from build123d import *

# Parameters (mm, degrees)
SKETCH1_W           = 7
SKETCH1_H           = 7
BOSS_EXTRUDE1_DEPTH = 3
FILLET1_R           = 1
BOSS_EXTRUDE2_DEPTH = 0.2
FILLET2_R           = 0.2


with BuildPart() as part:
    # Sketch1 → Boss-Extrude1 (new body)
    with BuildSketch(Plane(origin=(0, 0, 0), x_dir=(1, 0, 0), z_dir=(0, 1, 0))):
        Rectangle(SKETCH1_W, SKETCH1_H)
    extrude(amount=BOSS_EXTRUDE1_DEPTH)

    # Fillet1
    fillet1_edges = [part.edges().sort_by_distance(p)[0] for p in [
        (-3.5, 3, 0),
        (0, 3, 3.5),
        (3.5, 3, 0),
        (0, 3, -3.5),
        (3.5, 1.5, 3.5),
        (-3.5, 1.5, 3.5),
        (-3.5, 1.5, -3.5),
        (3.5, 1.5, -3.5),
    ]]
    fillet(fillet1_edges, radius=FILLET1_R)

    # Sketch2 → Boss-Extrude2 (add)
    with BuildSketch(Plane(origin=(0, 3, 0), x_dir=(1, 0, 0), z_dir=(0, 1, 0))):
        Polygon((0, 2), (-1.732050808, -1), (1.732050808, -1), align=None)
    extrude(amount=BOSS_EXTRUDE2_DEPTH)

    # Fillet2
    fillet2_edges = [part.edges().sort_by_distance(p)[0] for p in [
        (-0.866025404, 3.2, -0.5),
        (0.866025404, 3.2, -0.5),
        (0, 3.2, 1),
    ]]
    fillet(fillet2_edges, radius=FILLET2_R - 0.0001)  # a hair under: the kernel refuses the full size


solid = part.part
CAD build for the part. Positions are in the model's coordinates, mm. Round coordinates to 2 decimals unless told otherwise and drop trailing zeros. Loops run counter-clockwise (first coordinate to the right, second up) from the corner with the lowest first, then second, coordinate; pieces in that order, holes last.
(1) Wall check: line 1 along Y through (x, z) = (1, 2.5); line 2 along Y through (x, z) = (-1.25, 3); line 3 along Z through (x, y) = (2.75, 0.15). Give the ranges that are in metal, low to high.
(2) Cut at A-A (y = 1.05). Give the cut face in (x, z).
(3) Cut at C-C (x = 3). Give the cut face in (y, z), plus the area to 3 significant figures.
(4) Cut at B-B (z = 1.25). Give the cut face in (x, y).
(5) Cut at D-D (y = 2.55). Give the cut face in (x, z).
Findings below:
1. line 1: y = 0 to 3
1. line 2: y = 0 to 2.87
1. line 3: z = -3.47 to 3.47
2. outline: (-3.5, -2.5) arc R1 ccw to (-2.5, -3.5) - (2.5, -3.5) arc R1 ccw to (3.5, -2.5) - (3.5, 2.5) arc R1 ccw to (2.5, 3.5) - (-2.5, 3.5) arc R1 ccw to (-3.5, 2.5) - close
3. outline: (0, -3.37) - (2, -3.37) arc R0.87 ccw to (2.87, -2.5) - (2.87, 2.5) arc R0.87 ccw to (2, 3.37) - (0, 3.37) - close
3. area: 19.0 mm2
4. outline: (-3.5, 0) - (3.5, 0) - (3.5, 2) arc R1 ccw to (2.5, 3) - (-2.5, 3) arc R1 ccw to (-3.5, 2) - close
5. outline: (-3.34, -2.5) arc R0.84 ccw to (-2.5, -3.34) - (2.5, -3.34) arc R0.84 ccw to (3.34, -2.5) - (3.34, 2.5) arc R0.84 ccw to (2.5, 3.34) - (-2.5, 3.34) arc R0.84 ccw to (-3.34, 2.5) - close
